from build123d import *

# Parameters (mm, degrees)
SKETCH1_W      = 160
SKETCH1_H      = 70
EXTRUDE1_DEPTH = 3
SKETCH2_R      = 2
EXTRUDE2_DEPTH = 120
SKETCH3_R      = 1.5
EXTRUDE3_DEPTH = 10
SKETCH4_R      = 1.5
EXTRUDE4_DEPTH = 10
SKETCH5_R      = 1.5
EXTRUDE5_DEPTH = 10
SKETCH6_W      = 5
SKETCH6_H      = 10
EXTRUDE6_DEPTH = 5


with BuildPart() as part:
    # Sketch1 → Extrude1 (new body)
    with BuildSketch(Plane(origin=(0, 0, 0), x_dir=(1, 0, 0), z_dir=(0, 1, 0))):
        Rectangle(SKETCH1_W, SKETCH1_H)
    extrude(amount=EXTRUDE1_DEPTH)

    # Sketch2 → Extrude2 (cut)
    with BuildSketch(Plane(origin=(0, 3, 0), x_dir=(1, 0, 0), z_dir=(0, 1, 0))):
        with Locations(Location((-75, 30, 0), (0, 0, 270))):
            Circle(SKETCH2_R)
        with Locations(Location((-75, -30, 0), (0, 0, 270))):
            Circle(SKETCH2_R)
        with Locations(Location((75, -30, 0), (0, 0, 270))):
            Circle(SKETCH2_R)
        with Locations(Location((75, 30, 0), (0, 0, 270))):
            Circle(SKETCH2_R)
    extrude(amount=-EXTRUDE2_DEPTH, mode=Mode.SUBTRACT)

    # Sketch3 → Extrude3 (cut)
    with BuildSketch(Plane(origin=(0, 3, 0), x_dir=(1, 0, 0), z_dir=(0, 1, 0))):
        with Locations(Location((-59, 27, 0), (0, 0, 270))):
            Circle(SKETCH3_R)
        with Locations(Location((-59, -27, 0), (0, 0, 270))):
            Circle(SKETCH3_R)
        with Locations(Location((59, -27, 0), (0, 0, 270))):
            Circle(SKETCH3_R)
        with Locations(Location((59, 27, 0), (0, 0, 270))):
            Circle(SKETCH3_R)
    extrude(amount=-EXTRUDE3_DEPTH, mode=Mode.SUBTRACT)

    # Sketch4 → Extrude4 (cut)
    with BuildSketch(Plane(origin=(0, 3, 0), x_dir=(1, 0, 0), z_dir=(0, 1, 0))):
        with Locations(Location((-69.5, 12, 0), (0, 0, 270))):
            Circle(SKETCH4_R)
        with Locations(Location((-69.5, -12, 0), (0, 0, 270))):
            Circle(SKETCH4_R)
        with Locations(Location((69.5, -12, 0), (0, 0, 270))):
            Circle(SKETCH4_R)
        with Locations(Location((69.5, 12, 0), (0, 0, 270))):
            Circle(SKETCH4_R)
    extrude(amount=-EXTRUDE4_DEPTH, mode=Mode.SUBTRACT)

    # Sketch5 → Extrude5 (cut)
    with BuildSketch(Plane(origin=(0, 3, 0), x_dir=(1, 0, 0), z_dir=(0, 1, 0))):
        with Locations(Location((-42.5, 29, 0), (0, 0, 270))):
            Circle(SKETCH5_R)
        with Locations(Location((-42.5, -29, 0), (0, 0, 270))):
            Circle(SKETCH5_R)
        with Locations(Location((42.5, -29, 0), (0, 0, 270))):
            Circle(SKETCH5_R)
        with Locations(Location((42.5, 29, 0), (0, 0, 270))):
            Circle(SKETCH5_R)
    extrude(amount=-EXTRUDE5_DEPTH, mode=Mode.SUBTRACT)

    # Sketch6 → Extrude6 (cut)
    with BuildSketch(Plane.XZ):
        with Locations((-65.5, 0)):
            Rectangle(SKETCH6_W, SKETCH6_H)
    extrude(amount=-EXTRUDE6_DEPTH, mode=Mode.SUBTRACT)


solid = part.part
Here's how the part is built. I have some questions about the finished solid (model axes, mm). A direction names the side the tool comes from. Coordinates: 2 decimals unless noted, no trailing zeros. Write each loop counter-clockwise with the first axis right and the second up, starting at its lowest first coordinate (ties: lowest second). Pieces come first, ordered by that corner, then holes.
1) I'm going to push a flat-ended pin straight in: pin 1 (1.8 mm diameter, centred on x = 59, z = -27, fed in from -Y). Where does the tip first touch, or does it pass through?
Filled in:
pin 1: passes through
2) Which directions (+Z, -Z, +X, -X, +Y, -Y) give clear straight access to the entire face, cutting with the end or side of a thin tool? Please do faces 5 (the face through (-1, 3, 0)), 6 (the face through (-66, 1, -5)).
Filled in:
face 5: +Z, -Z, +X, -X, +Y
face 6: +Y, -Y
3) If we section it at B-B (z = -12): List the corners of the cut face in (x, y) for me.
Filled in:
outline: (-80, 0) - (-71, 0) - (-71, 3) - (-80, 3) - close; (-68, 0) - (68, 0) - (68, 3) - (-68, 3) - close; (71, 0) - (80, 0) - (80, 3) - (71, 3) - close
4) Thinking about a two-plate mould opening in X: for faces 1 (the face through (-80, 1, 0)), 2 (the face through (-63, 1, 0)), 3 (the face through (-43.4, 1.5, 27.8)), 4 (the face through (-1, 0, 0)), which applies, +X half, -X half, draft (parallel to the pull), parting line (faces both ways), or undercut?
Filled in:
face 1: -X half
face 2: undercut
face 3: undercut
face 4: draft
5) If we section it at C-C (y = 0.9): Count the separate pieces of the cut face and the enclosed holes in it, plus the area to 3 significant figures.
Filled in:
separate pieces: 1
enclosed holes: 17
area: 11,000 mm2
6) If we section it at A-A (x = -59): List the corners of the cut face in (y, z) for me, plus the area to 3 significant figures.
Filled in:
outline: (0, -35) - (3, -35) - (3, -28.5) - (0, -28.5) - close; (0, -25.5) - (3, -25.5) - (3, 25.5) - (0, 25.5) - close; (0, 28.5) - (3, 28.5) - (3, 35) - (0, 35) - close
area: 192 mm2
7) If I drill on line 1 (Z direction, x = -64, y = 2.1); line 2 (X direction, y = 1.2, z = 27); line 3 (X direction, y = 0.9, z = 12), over which ranges is the centre line in solid material (lowest first)?
Filled in:
line 1: z = -35 to -5, 5 to 35
line 2: x = -80 to -60.5, -57.5 to 57.5, 60.5 to 80
line 3: x = -80 to -71, -68 to 68, 71 to 80
